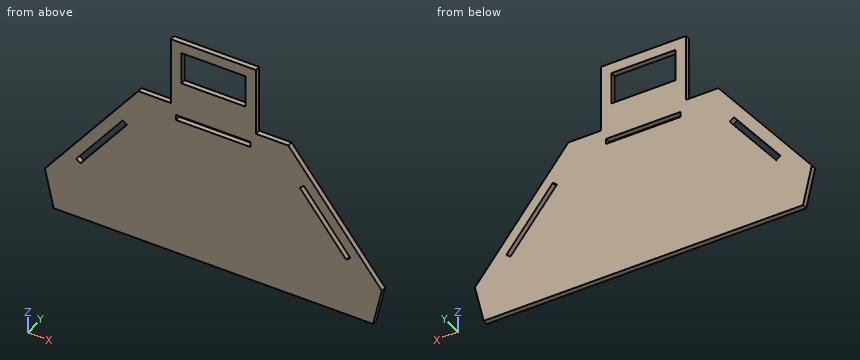
from build123d import *

# Parameters (mm, degrees)
F0_W     = 70
F0_H     = 5
F1_DEPTH = 5


with BuildPart() as f1:
    # F0 (on Front) → F1 (new body)
    with BuildSketch(Plane.XZ):
        Polygon((-40, 146.239187), (-70.425081, 146.239187), (-158.24372, 36.118096), (-150, 0), (150, 0), (158.24372, 36.118096), (70.425081, 146.239187), (40, 146.239187), (40, 209.417821), (1.491508, 209.417821), (-40, 209.417821), align=None)
        Polygon((-81.164699, 108.714), (-124.808985, 53.985796), (-128.718142, 57.103245), (-85.073856, 111.831449), align=None, mode=Mode.SUBTRACT)
        Polygon((128.718142, 57.103245), (124.808985, 53.985796), (81.164699, 108.714), (85.073856, 111.831449), align=None, mode=Mode.SUBTRACT)
        with Locations((0, 133.739187)):
            Rectangle(F0_W, F0_H, mode=Mode.SUBTRACT)
        Polygon((-30, 199.417821), (0, 199.417821), (30, 199.417821), (30, 169.417821), (-30, 169.417821), align=None, mode=Mode.SUBTRACT)
    extrude(amount=F1_DEPTH)


solid = f1.part
Read the model definition and answer for the solid it produces. Units are mm, in the model's axes. Give positions to 0.01 mm unless a question says otherwise; leave off trailing zeros. Write each loop counter-clockwise with the first axis right and the second up, starting at its lowest first coordinate (ties: lowest second). Pieces come first, ordered by that corner, then holes. Notation, with made-up numbers: (17.5, -38.75) - (62.5, -38.75) arc R12 ccw to (62.5, -33.75) - close; hole circle Ø7 at (3, -15.75). An arc over 180 degrees is marked (long way). Use CSV: the item, a comma, the result in double quotes. Start each with the question number.
(1) Find section C-C (x = 24). Give the vertices of the cut face in (y, z).
(2) Find section A-A (z = 183). Give the vertices of the cut face in (x, y).
(3) Consider line 1 along Z through (x, y) = (-13, -0.35); line 2 along X through (y, z) = (-3.75, 87.5); line 3 along X through (y, z) = (-0.6, 189.5). Determine where each line is inside the solid, lowest interval first.
(4) Find section B-B (y = -4). Give the vertices of the cut face in (x, z).
(5) Find section D-D (x = 114). Give the vertices of the cut face in (y, z), plus the area to 3 significant figures.
(6) Given P1, Ø1.5, axis at x = -116, y = -1.5, coming from the +Z side; P2, Ø2, axis at y = -3.5, z = 162.5, coming from the +X side; P3, Ø1.5, axis at y = -1.5, z = 65.5, coming from the +X side, each flat-ended and moving along its own axis, determine where each tip first touches the part or whether it passes through.
Findings below:
1,outline,"(-5, 0) - (0, 0) - (0, 131.24) - (-5, 131.24) - close; (-5, 136.24) - (0, 136.24) - (0, 169.42) - (-5, 169.42) - close; (-5, 199.42) - (0, 199.42) - (0, 209.42) - (-5, 209.42) - close"
2,outline,"(-40, -5) - (-30, -5) - (-30, 0) - (-40, 0) - close; (30, -5) - (40, -5) - (40, 0) - (30, 0) - close"
3,line 1,"0 to 131.24, 136.24 to 169.42, 199.42 to 209.42"
3,line 2,"-117.27 to -104.48, -98.08 to 98.08, 104.48 to 117.27"
3,line 3,"-40 to -30, 30 to 40"
4,outline,"(-158.24, 36.12) - (-150, 0) - (150, 0) - (158.24, 36.12) - (70.43, 146.24) - (40, 146.24) - (40, 209.42) - (-40, 209.42) - (-40, 146.24) - (-70.43, 146.24) - close; hole (-128.72, 57.1) - (-124.81, 53.99) - (-81.16, 108.71) - (-85.07, 111.83) - close; hole (-35, 131.24) - (35, 131.24) - (35, 136.24) - (-35, 136.24) - close; hole (-30, 169.42) - (30, 169.42) - (30, 199.42) - (-30, 199.42) - close; hole (81.16, 108.71) - (124.81, 53.99) - (128.72, 57.1) - (85.07, 111.83) - close"
5,outline,"(-5, 0) - (0, 0) - (0, 67.54) - (-5, 67.54) - close; (-5, 75.56) - (0, 75.56) - (0, 91.6) - (-5, 91.6) - close"
5,area,"418 mm2"
6,P1,"z = 90.03"
6,P2,"x = 40"
6,P3,"x = 135.41"
